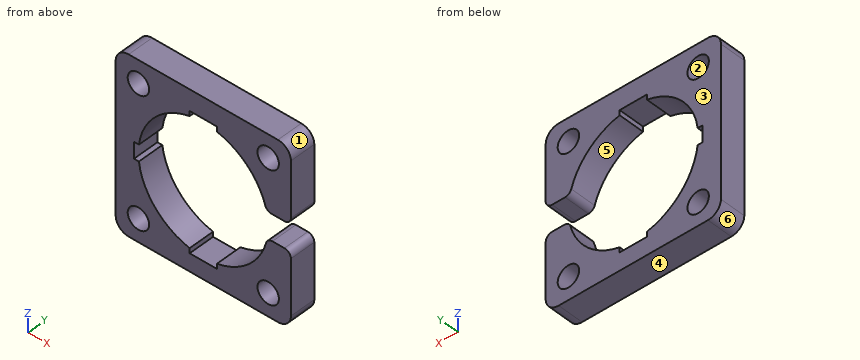
from build123d import *

# Parameters (mm, degrees)
SKETCH1_W           = 27
SKETCH1_H           = 27
SKETCH1_R           = 1.65
BOSS_EXTRUDE1_DEPTH = 4
CUT_EXTRUDE1_DEPTH  = 20.506409203
FILLET2_R           = 2
SKETCH5_W           = 14.325764552
SKETCH5_H           = 4
CUT_EXTRUDE2_DEPTH  = 20.506409203
FILLET3_R           = 1


with BuildPart() as part:
    # Sketch1 → Boss-Extrude1 (new body)
    with BuildSketch(Plane(origin=(0, 0, 0), x_dir=(1, 0, 0), z_dir=(0, 1, 0))):
        Rectangle(SKETCH1_W, SKETCH1_H)
        with Locations(Location((10, 10, 0), (0, 0, 270))):
            Circle(SKETCH1_R, mode=Mode.SUBTRACT)
        with Locations(Location((10, -10, 0), (0, 0, 270))):
            Circle(SKETCH1_R, mode=Mode.SUBTRACT)
        with Locations(Location((-10, -10, 0), (0, 0, 270))):
            Circle(SKETCH1_R, mode=Mode.SUBTRACT)
        with Locations(Location((-10, 10, 0), (0, 0, 270))):
            Circle(SKETCH1_R, mode=Mode.SUBTRACT)
    extrude(amount=BOSS_EXTRUDE1_DEPTH)

    # Sketch2 → Cut-Extrude1 (cut, through all)
    with BuildSketch(Plane(origin=(0, 4, 0), x_dir=(1, 0, 0), z_dir=(0, 1, 0))):
        with BuildLine():
            Line((-9.921567416, 1.5), (-10.677078252, 1.5))
            Line((-10.677078252, 1.5), (-10.677078252, -1))
            Line((-10.677078252, -1), (-9.921567416, -1))
            ThreePointArc((-9.921567416, -1), (-7.36932915, -6.509658858), (-2.1, -9.527013859))
            Line((-2.1, -9.527013859), (-2.1, -10.292888598))
            Line((-2.1, -10.292888598), (2.1, -10.292888598))
            Line((2.1, -10.292888598), (2.1, -9.527013859))
            ThreePointArc((2.1, -9.527013859), (7.36932915, -6.509658858), (9.921567416, -1))
            Line((9.921567416, -1), (10.677078252, -1))
            Line((10.677078252, -1), (10.677078252, 1.5))
            Line((10.677078252, 1.5), (9.921567416, 1.5))
            ThreePointArc((9.921567416, 1.5), (7.36932915, 7.009658858), (2.1, 10.027013859))
            Line((2.1, 10.027013859), (2.1, 10.792888598))
            Line((2.1, 10.792888598), (-2.1, 10.792888598))
            Line((-2.1, 10.792888598), (-2.1, 10.027013859))
            ThreePointArc((-2.1, 10.027013859), (-7.36932915, 7.009658858), (-9.921567416, 1.5))
        make_face()
    extrude(amount=-CUT_EXTRUDE1_DEPTH, mode=Mode.SUBTRACT)

    # Fillet2
    fillet2_edges = [part.edges().sort_by_distance(p)[0] for p in [
        (13.5, 2, 13.5),
        (-13.5, 2, 13.5),
        (-13.5, 2, -13.5),
        (13.5, 2, -13.5),
    ]]
    fillet(fillet2_edges, radius=FILLET2_R)

    # Sketch5 → Cut-Extrude2 (cut, through all)
    with BuildSketch(Plane(origin=(0, 4, 0), x_dir=(1, 0, 0), z_dir=(0, 1, 0))):
        with Locations((10.779204511, 0)):
            Rectangle(SKETCH5_W, SKETCH5_H)
    extrude(amount=-CUT_EXTRUDE2_DEPTH, mode=Mode.SUBTRACT)

    # Fillet3
    fillet3_edges = [part.edges().sort_by_distance(p)[0] for p in [
        (9.743587635, 2, 2),
        (9.845684334, 2, -2),
        (13.5, 2, -2),
        (13.5, 2, 2),
    ]]
    fillet(fillet3_edges, radius=FILLET3_R)


solid = part.part
Model file for the job. Use its own axes, mm. Face numbers are marked on the shaded views. A direction names the side the tool comes from. Give positions to 0.01 mm unless a question says otherwise; leave off trailing zeros. Loops run counter-clockwise (first coordinate to the right, second up) from the corner with the lowest first, then second, coordinate; pieces in that order, holes last.
Item 1: Slice it at D-D (x = 11). Write the cut outline in (y, z).
Check values:
outline: (0, -13.5) - (4, -13.5) - (4, -11.31) - (0, -11.31) - close; (0, -8.69) - (4, -8.69) - (4, -2) - (0, -2) - close; (0, 2) - (4, 2) - (4, 8.69) - (0, 8.69) - close; (0, 11.31) - (4, 11.31) - (4, 13.5) - (0, 13.5) - close
Item 2: Slice it at C-C (x = -5). Write the cut outline in (y, z), plus the area to 3 significant figures.
Check values:
outline: (0, -13.5) - (4, -13.5) - (4, -8.91) - (0, -8.91) - close; (0, 8.41) - (4, 8.41) - (4, 13.5) - (0, 13.5) - close
area: 38.7 mm2
Item 3: Slice it at A-A (y = 3.1). Give the number of separate pieces and of enclosed holes in the cut face, plus the area to 3 significant figures.
Check values:
separate pieces: 1
enclosed holes: 4
area: 355 mm2
Item 4: Drill centre lines: line 1 along X through (y, z) = (2.35, 10); line 2 along Z through (x, y) = (0.5, 3.3); line 3 along Z through (x, y) = (9.75, 3.2). Where is each one in solid material? Low to high.
Check values:
line 1: x = -13.5 to -11.65, -8.35 to -2.1, 2.1 to 8.35, 11.65 to 13.5
line 2: z = -13.5 to -10.79, 10.29 to 13.5
line 3: z = -13.5 to -11.63, -8.37 to -2.57, 2.35 to 8.37, 11.63 to 13.5
Item 5: Drop a flat-ended pin along its axis: P1, Ø1.2, axis at y = 1, z = 0.5, coming from the +X side. Give the stop position or say it passes through.
Check values:
P1: stops at x = -9.91
Item 6: Mould opens along Z. For the marked faces 1, 2, 3 and 4 say: +Z half, -Z half, draft (parallel to the pull), parting line (faces both ways), or undercut.
Check values:
face 1: +Z half
face 2: undercut
face 3: draft
face 4: -Z half
Item 7: Which spindle directions (+Z, -Z, +X, -X, +Y, -Y) get a long thin tool onto all of the face, cutting with end or side? Do the marked faces 5 and 6. Say none if no direction does.
Check values:
face 5: +Y, -Y
face 6: -Z, -X, +Y, -Y
Item 8: Slice it at B-B (z = -6). Write the cut outline in (x, y), plus the area to 3 significant figures.
Check values:
outline: (-13.5, 0) - (-8.18, 0) - (-8.18, 4) - (-13.5, 4) - close; (8.18, 0) - (13.5, 0) - (13.5, 4) - (8.18, 4) - close
area: 42.5 mm2
